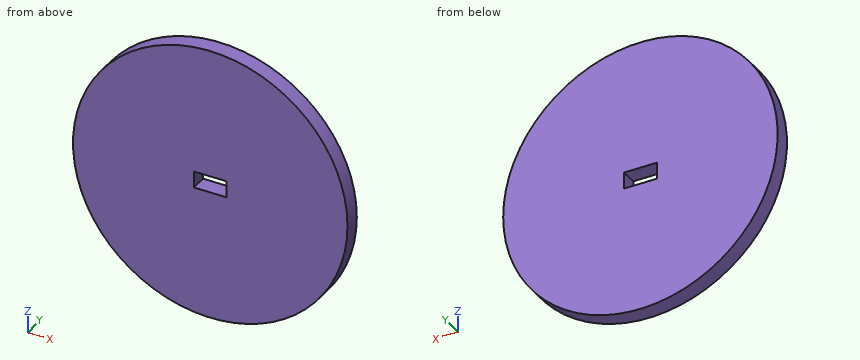
```python
from build123d import *

# Parameters (mm, degrees)
SKETCH_1_R          = 25
EXTRUDE_1_DEPTH     = 3
SKETCH_2_W          = 6
SKETCH_2_H          = 3
CUT_EXTRUDE_2_DEPTH = 11


with BuildPart() as part:
    # 草图1 → 凸台-拉伸1 (new body)
    with BuildSketch(Plane(origin=(0, 0, 0), x_dir=(1, 0, 0), z_dir=(0, 1, 0))):
        Circle(SKETCH_1_R)
    extrude(amount=EXTRUDE_1_DEPTH)

    # 草图2 → 切除-拉伸2 (cut)
    with BuildSketch(Plane(origin=(0, 3, 0), x_dir=(1, 0, 0), z_dir=(0, 1, 0))):
        Rectangle(SKETCH_2_W, SKETCH_2_H)
    extrude(amount=-CUT_EXTRUDE_2_DEPTH, mode=Mode.SUBTRACT)


solid = part.part
```
The model under review builds one solid part; all positions refer to its coordinate system, in mm. Round coordinates to 2 decimals unless told otherwise and drop trailing zeros. Order: outer loops, then holes, each group sorted by start corner. A loop starts at its lowest first (then second) coordinate and runs counter-clockwise, first axis right, second up. Notation, with made-up numbers: M 18,64 L 45,64 A19 ccw 45,84 Z; hole C -36.75,-3.75 d1. An arc over 180 degrees is marked long. Use a Markdown table: item, result.
1) Insertion check: pin 1 (1.5 mm diameter, centred on x = -7.5, y = 1, fed in from -Z); pin 2 (0.9 mm diameter, centred on x = 0, y = 1.5, fed in from -Z); pin 3 (1.5 mm diameter, centred on x = -1, y = 1, fed in from +Z). Each pin has a flat end and moves straight along its axis. Give the tip position at first contact, or say it passes through.
Report:
| item | result |
|---|---|
| pin 1 | z = -24.07 |
| pin 2 | z = -25 |
| pin 3 | z = 25 |
2) Wall thickness on line 1 along Z through (x, y) = (-0.5, 2.5) (3 decimals); line 2 along X through (y, z) = (1.45, -16); line 3 along X through (y, z) = (2.3, -11.5): over which ranges is each line inside the solid? List them lowest first. Write a range as [from, to].
Report:
| item | result |
|---|---|
| line 1 | [-24.995, -1.5], [1.5, 24.995] |
| line 2 | [-19.21, 19.21] |
| line 3 | [-22.2, 22.2] |
3) Consider section B-B (x = 0). Write out the cut boundary in (y, z), then the cut area to 3 significant figures.
Report:
| item | result |
|---|---|
| outline | M 0,-25 L 3,-25 L 3,-1.5 L 0,-1.5 Z; M 0,1.5 L 3,1.5 L 3,25 L 0,25 Z |
| area | 141 mm^2 |
4) Consider section C-C (y = 0.95). Write out the cut boundary in (x, z).
Report:
| item | result |
|---|---|
| outline | C 0,0 d50; hole M -3,-1.5 L 3,-1.5 L 3,1.5 L -3,1.5 Z |
5) Consider section A-A (z = 0). Write out the cut boundary in (x, y), then the cut area to 3 significant figures.
Report:
| item | result |
|---|---|
| outline | M -25,0 L -3,0 L -3,3 L -25,3 Z; M 3,0 L 25,0 L 25,3 L 3,3 Z |
| area | 132 mm^2 |
6) Consider section D-D (z = 11). Write out the cut boundary in (x, y), then the cut area to 3 significant figures.
Report:
| item | result |
|---|---|
| outline | M -22.45,0 L 22.45,0 L 22.45,3 L -22.45,3 Z |
| area | 135 mm^2 |
